Model file for the job. Use its own axes, mm. Round coordinates to 2 decimals unless told otherwise and drop trailing zeros. Loops run counter-clockwise (first coordinate to the right, second up) from the corner with the lowest first, then second, coordinate; pieces in that order, holes last. Notation, with made-up numbers: M 69,-11 L 86,-11 A17 ccw 86,13 Z; hole C 26,-14.5 d2. An arc over 180 degrees is marked long. Use a Markdown table: item, result. Add a question column.
Item 1: Saw through at B-B on y = 1.3. Give the number of separate pieces and of enclosed holes in the cut face, then the cut area to 3 significant figures.
Item 2: Wall check: L1, parallel to X at y = 1.3, z = -29.72; L2, parallel to X at y = 0.55, z = 64; L3, parallel to Z at x = 16, y = 1.2. Give the ranges that are in metal, low to high. Write a range as from..to.
Item 3: Saw through at A-A on z = -50. Write the cut outline in (x, y), then the cut area to 3 significant figures.
Item 4: Two-plate mould, pull along Z, no slides. Class faces 1 (the cylindrical face through (0.53, 1.01, -61.99)), 2 (the flat face through (-4, 2, -2)): +Z half, -Z half, draft (parallel to the pull), parting line (faces both ways), or undercut.
```python
from build123d import *

# Parameters (mm, degrees)
SKETCH1_W           = 508
SKETCH1_H           = 296
BOSS_EXTRUDE1_DEPTH = 2
SKETCH2_R           = 12
SKETCH2_R_2         = 2.65
SKETCH2_R_3         = 2.9
SKETCH2_W           = 65
SKETCH2_H           = 36
CUT_EXTRUDE1_DEPTH  = 10
SKETCH4_R           = 3.4
CUT_EXTRUDE2_DEPTH  = 10


with BuildPart() as part:
    # Sketch1 → Boss-Extrude1 (new body)
    with BuildSketch(Plane(origin=(0, 0, 0), x_dir=(1, 0, 0), z_dir=(0, 1, 0))):
        Rectangle(SKETCH1_W, SKETCH1_H)
    extrude(amount=BOSS_EXTRUDE1_DEPTH)

    # Sketch2 → Cut-Extrude1 (cut)
    with BuildSketch(Plane(origin=(0, 2, 0), x_dir=(1, 0, 0), z_dir=(0, 1, 0))):
        with Locations(Location((0, 50, 0), (0, 0, 270))):
            Circle(SKETCH2_R)
        with Locations(Location((-20.28, 70.28, 0), (0, 0, 270))):
            Circle(SKETCH2_R_2)
        with Locations(Location((-20.28, 29.72, 0), (0, 0, 90))):
            Circle(SKETCH2_R_2)
        with Locations(Location((20.28, 29.72, 0), (0, 0, 270))):
            Circle(SKETCH2_R_2)
        with Locations(Location((20.28, 70.28, 0), (0, 0, 90))):
            Circle(SKETCH2_R_2)
        with Locations(Location((41.5, -32, 0), (0, 0, 270))):
            Circle(SKETCH2_R_3)
        with Locations(Location((41.5, -64, 0), (0, 0, 270))):
            Circle(SKETCH2_R_3)
        with Locations(Location((-41.5, -64, 0), (0, 0, 270))):
            Circle(SKETCH2_R_3)
        with Locations(Location((-41.5, -32, 0), (0, 0, 270))):
            Circle(SKETCH2_R_3)
        with Locations((0, -48)):
            Rectangle(SKETCH2_W, SKETCH2_H)
    extrude(amount=-CUT_EXTRUDE1_DEPTH, mode=Mode.SUBTRACT)

    # Sketch4 → Cut-Extrude2 (cut)
    with BuildSketch(Plane.XZ):
        with Locations(Location((-239, 133, 0), (0, 0, 270))):
            Circle(SKETCH4_R)
        with Locations(Location((239, 133, 0), (0, 0, 270))):
            Circle(SKETCH4_R)
        with Locations(Location((-239, -133, 0), (0, 0, 270))):
            Circle(SKETCH4_R)
        with Locations(Location((239, -133, 0), (0, 0, 270))):
            Circle(SKETCH4_R)
    extrude(amount=-CUT_EXTRUDE2_DEPTH, mode=Mode.SUBTRACT)


solid = part.part
```
Entries:
| question | item | result |
|---|---|---|
| 1 | separate pieces | 1 |
| 1 | enclosed holes | 14 |
| 1 | area | 147,000 mm2 |
| 2 | L1 | -254..-22.93, -17.63..17.63, 22.93..254 |
| 2 | L2 | -254..-44.4, -38.6..-32.5, 32.5..38.6, 44.4..254 |
| 2 | L3 | -148..30, 66..148 |
| 3 | outline | M -254,0 L -12,0 L -12,2 L -254,2 Z; M 12,0 L 254,0 L 254,2 L 12,2 Z |
| 3 | area | 968 mm2 |
| 4 | face 1 | undercut |
| 4 | face 2 | draft |
